```python
from build123d import *

# Parameters (mm, degrees)
EXTRUDE_1_DEPTH     = 5
SKETCH_2_W          = 20.2
SKETCH_2_H          = 8
CUT_EXTRUDE_1_DEPTH = 6
SKETCH_3_R          = 1.15
EXTRUDE_2_DEPTH     = 6
CHAMFER_1_SIZE      = 5
SKETCH_4_R          = 3
CUT_EXTRUDE_2_DEPTH = 6
SKETCH_5_R          = 1.6
CUT_EXTRUDE_3_DEPTH = 5


with BuildPart() as part:
    # 草图1 → 凸台-拉伸1 (new body, symmetric)
    with BuildSketch(Plane(origin=(0, 0, 0), x_dir=(0, 0, -1), z_dir=(1, 0, 0))):
        Polygon((0, 0), (30, 0), (30, 35), (45, 35), (45, 39), (25, 39), (25, 8), (0, 8), align=None)
    extrude(amount=EXTRUDE_1_DEPTH, both=True)

    # 草图2 → 切除-拉伸1 (cut)
    with BuildSketch(Plane.ZY.offset(5)):
        with Locations((-12.5, 4)):
            Rectangle(SKETCH_2_W, SKETCH_2_H)
    extrude(amount=-CUT_EXTRUDE_1_DEPTH, mode=Mode.SUBTRACT)

    # 草图3 → 凸台-拉伸2 (add)
    with BuildSketch(Plane.ZY.offset(-1)):
        with Locations((-17.25, 2.5)):
            Circle(SKETCH_3_R)
        with Locations((-7.75, 2.5)):
            Circle(SKETCH_3_R)
    extrude(amount=EXTRUDE_2_DEPTH)

    # 倒角1
    chamfer_1_edges = [part.edges().sort_by_distance(p)[0] for p in [
        (0, 8, -25),
        (0, 35, -30),
    ]]
    chamfer(chamfer_1_edges, length=CHAMFER_1_SIZE)

    # 草图4 → 切除-拉伸2 (cut)
    with BuildSketch(Plane.XZ.offset(-35)):
        with Locations((0, -35)):
            Circle(SKETCH_4_R)
    extrude(amount=CUT_EXTRUDE_2_DEPTH, mode=Mode.SUBTRACT)

    # 草图5 → 切除-拉伸3 (cut, through all)
    with BuildSketch(Plane.XZ.offset(-35)):
        with Locations((0, -35)):
            Circle(SKETCH_5_R)
    extrude(amount=-CUT_EXTRUDE_3_DEPTH, mode=Mode.SUBTRACT)


solid = part.part
```
Work out the finished part from the listing and answer in its coordinate system (mm). A direction names the side the tool comes from. Coordinates: 2 decimals unless noted, no trailing zeros. Write each loop counter-clockwise with the first axis right and the second up, starting at its lowest first coordinate (ties: lowest second). Pieces come first, ordered by that corner, then holes. Notation, with made-up numbers: (40, 27) - (82, 27) arc R32 ccw to (82, 57) - close; hole circle Ø6 at (-14, 52). An arc over 180 degrees is marked (long way). Answer as a JSON object with one key per item and string values.
Q1. Find section B-B (x = 0). Write down the section's boundary in (y, z).
Results list:
{"outline": "(0, -30) - (30, -30) - (32, -32) - (35, -32) - (35, -33.4) - (39, -33.4) - (39, -25) - (13, -25) - (10.6, -22.6) - (0, -22.6) - close; (0, -2.4) - (8, -2.4) - (8, 0) - (0, 0) - close; circle Ø2.3 at (2.5, -17.25); circle Ø2.3 at (2.5, -7.75); (35, -45) - (39, -45) - (39, -36.6) - (35, -36.6) - close"}
Q2. Which of the six approach directions +Z, -Z, +X, -X, +Y, -Y give full straight-line access (tool end or side, diameter ignored) to faces 4 (the flat face through (0, 4, 0)), 5 (the flat face through (-2, 5, -22.6)), 6 (the cylindrical face through (-1.96, 2.55, -18.4)), 7 (the flat face through (2, 8, -10)), 8 (the flat face through (0, 15, -30))?
Results list:
{"face 4": "+Z, +X, -X, +Y, -Y", "face 5": "-X, +Y, -Y", "face 6": "-X", "face 7": "+Z, +X, -X, +Y", "face 8": "-Z, +X, -X, -Y"}
Q3. Consider L1, parallel to Z at x = 0, y = 37.4; L2, parallel to Z at x = -3.25, y = 20; L3, parallel to Y at x = -3.5, z = -39. Determine where each line is inside the solid, lowest interval first. Write a range as from..to.
Results list:
{"L1": "z = -45..-36.6, -33.4..-25", "L2": "z = -30..-25", "L3": "y = 35..39"}
Q4. Given pin 1 Ø5 at (x, z) = (2, -16) entering from +Y; pin 2 Ø3 at (x, y) = (-1.5, 17.5) entering from +Z; pin 3 Ø4 at (x, y) = (-3.5, 31.5) entering from -Z; pin 4 Ø8.5 at (y, z) = (4.5, -10) entering from -X, each flat-ended and moving along its own axis, determine where each tip first touches the part or whether it passes through.
Results list:
{"pin 1": "stops at y = 8", "pin 2": "stops at z = -25", "pin 3": "stops at z = -33.5", "pin 4": "stops at x = -5"}
Q5. Find section A-A (y = 36). Write down the section's boundary in (x, z), plus the area to 3 significant figures.
Results list:
{"outline": "(-5, -45) - (5, -45) - (5, -25) - (-5, -25) - close; hole circle Ø3.2 at (0, -35)", "area": "192 mm^2"}
Q6. Find section D-D (y = 7). Write down the section's boundary in (x, z).
Results list:
{"outline": "(-5, -30) - (5, -30) - (5, 0) - (-5, 0) - (-5, -2.4) - (1, -2.4) - (1, -22.6) - (-5, -22.6) - close"}
Q7. Find section C-C (z = -7.75). Write down the section's boundary in (x, y).
Results list:
{"outline": "(-5, 1.35) - (1, 1.35) - (1, 0) - (5, 0) - (5, 8) - (1, 8) - (1, 3.65) - (-5, 3.65) - close"}
Q8. For a pull along X with two mould halves and no side action, classify faces 1 (the cylindrical face through (0, 34, -32)), 2 (the flat face through (-2, 4, -2.4)), 3 (the flat face through (-5, 4, -1)) as pulls with the +X half, pulls with the -X half, needs draft (parallel to the pull), parting line crosses it, or undercut.
Results list:
{"face 1": "undercut", "face 2": "needs draft", "face 3": "pulls with the -X half"}
